Verification items for the finished model (mm, model axes). A direction names the side the tool comes from. Coordinates: 2 decimals unless noted, no trailing zeros. Write each loop counter-clockwise with the first axis right and the second up, starting at its lowest first coordinate (ties: lowest second). Pieces come first, ordered by that corner, then holes. Notation, with made-up numbers: M 50,-0.5 L 108,-0.5 A18 ccw 108,5.5 Z; hole C 88.5,42.5 d7. An arc over 180 degrees is marked long. One line per item, written item: value.
```python
from build123d import *

# Parameters (mm, degrees)
F1_DEPTH    = 15
F2_T1_DEPTH = 15


# Not quite as in the source:
# - a fillet or chamfer that OpenCascade refuses, or shapes differently, is made with other operations: its cross-section is extruded or revolved along the edge and cut away or added


with BuildPart() as f1:
    # F0 (on Top) → F1 (new body)
    with BuildSketch(Plane.XY):
        with BuildLine():
            ThreePointArc((-40, 41.475575803), (-39.267766953, 43.243342756), (-37.5, 43.975575803))
            Line((-37.5, 43.975575803), (0, 43.975575803))
            Line((0, 43.975575803), (0, 47.775575803))
            Line((0, 47.775575803), (-37.5, 47.775575803))
            ThreePointArc((-37.5, 47.775575803), (-41.9618437893, 45.9274195923), (-43.81, 41.465575803))
            Line((-43.81, 41.465575803), (-43.81, 36.475575803))
            Line((-43.81, 36.475575803), (-43.81, -27.529513372))
            Line((-43.81, -27.529513372), (-43.81, -37.104424197))
            Line((-43.81, -37.104424197), (-48.4908909885, -28.7516895034))
            Line((-48.4908909885, -28.7516895034), (-56.369773679, -14.6923540142))
            Line((-56.369773679, -14.6923540142), (-56.7601447269, -13.9957631722))
            ThreePointArc((-56.7601447269, -13.9957631722), (-57.782169231, -13.1905372922), (-59.0742303685, -13.3438370694))
            Line((-59.0742303685, -13.3438370694), (-59.2530634296, -13.4440555122))
            Line((-59.2530634296, -13.4440555122), (-59.4318964906, -13.5442739549))
            ThreePointArc((-59.4318964906, -13.5442739549), (-60.2371223706, -14.566298459), (-60.0838225934, -15.8583595965))
            Line((-60.0838225934, -15.8583595965), (-59.6934515455, -16.5549504386))
            Line((-59.6934515455, -16.5549504386), (-47.1336778665, -38.9670206213))
            ThreePointArc((-47.1336778665, -38.9670206213), (-42.8474805641, -40.7908393032), (-40, -37.104424197))
            Line((-40, -37.104424197), (-40, 30.165575803))
            Line((-40, 30.165575803), (-37.5, 30.165575803))
            Line((-37.5, 30.165575803), (-36.5, 30.165575803))
            Line((-36.5, 30.165575803), (-36.5, 33.975575803))
            Line((-36.5, 33.975575803), (-37.5, 33.975575803))
            ThreePointArc((-37.5, 33.975575803), (-39.267766953, 34.7078088501), (-40, 36.475575803))
            Line((-40, 36.475575803), (-40, 41.475575803))
        make_face()
    extrude(amount=F1_DEPTH)

    # F2: fillet of radius 7 on 1 edges, made by hand

    # F2_s2 → F2_t1 (join)
    with BuildSketch(Plane.XY):
        with BuildLine():
            add(Edge.make_bspline(
                [(-56.7906958843, -13.9434544078), (-43.81, -35.286127782), (-43.81, -10.30597221)],
                knots=[0, 0, 0, 1, 1, 1], degree=2, weights=[1, 1, 1]))
            Line((-43.81, -10.30597221), (-43.11, -10.30597221))
            Line((-43.11, -10.30597221), (-43.11, -37.104424197))
            Line((-43.11, -37.104424197), (-44.4206494768, -37.4466335138))
            ThreePointArc((-44.4206494768, -37.4466335138), (-57.3707942037, -14.337972489), (-57.3887654728, -14.3072026276))
            Line((-57.3887654728, -14.3072026276), (-56.7906958843, -13.9434544078))
        make_face()
    extrude(amount=F2_T1_DEPTH)

    # F3: F1 across face


with BuildPart() as f1_1:
    add(f1.part)
    add(f1.part.mirror(Plane(origin=(0, 45.875575803, 7.5), x_dir=(0, 1, 0), z_dir=(1, 0, 0))))


solid = f1_1.part
```
Item 1: Scan lines: line 1 (X direction, y = -10.5, z = 9); line 2 (X direction, y = -20, z = 13.5); line 3 (Y direction, x = 3.5, z = 9). Record each from-to range of solid material in increasing order.
The answers:
line 1: x = -43.81 to -40, 40 to 43.81
line 2: x = -57.76 to -52.64, -44.65 to -40, 40 to 44.65, 52.64 to 57.76
line 3: y = 43.98 to 47.78
Item 2: Access from +Z, -Z, +X, -X, +Y, -Y to the whole of each face (thin tool, end or side, straight path). Record for faces 4 (the face through (43.81, 16, 7)), 5 (the face through (-40, 39, 7)), 6 (the face through (-36.5, 32, 7)).
The answers:
face 4: +Z, -Z, +X, +Y
face 5: +Z, -Z
face 6: +Z, -Z, -Y
Item 3: Cross-section at B-B, the plane x = 1. Enter the section's corners in (y, z).
The answers:
outline: M 43.98,0 L 47.78,0 L 47.78,15 L 43.98,15 Z
Item 4: Go/stop test with flat-tipped pins: P1, Ø5.5, axis at y = 39, z = 4, coming from the +X side; P2, Ø7.5, axis at y = -11.5, z = 9, coming from the +X side; P3, Ø5.5, axis at y = 40, z = 10, coming from the -X side; P4, Ø4, axis at x = -11, z = 8, coming from the -Y side. Record where each tip stops, or that it passes through.
The answers:
P1: stops at x = 43.81
P2: stops at x = 60.3
P3: stops at x = -43.81
P4: stops at y = 43.98
Item 5: Draft check along X on faces 1 (the face through (-43.81, 16, 7)), 2 (the face through (-57.79, -13.19, 7.4)), 3 (the face through (-40.5, 3.6, 15)). Enter one of: released by +X, released by -X, zero draft, split by the parting line, or undercut.
The answers:
face 1: released by -X
face 2: undercut
face 3: zero draft
Item 6: Cross-section at A-A, the plane y = -7. Enter the section's corners in (x, z), and give its area (3 significant figures).
The answers:
outline: M -43.81,0 L -40,0 L -40,15 L -43.81,15 Z; M 40,0 L 43.81,0 L 43.81,15 L 40,15 Z
area: 114 mm²
